CAD build for the part. Positions are in the model's coordinates, mm. Face numbers are marked on the shaded views. Give positions to 0.01 mm unless a question says otherwise; leave off trailing zeros. Loops run counter-clockwise (first coordinate to the right, second up) from the corner with the lowest first, then second, coordinate; pieces in that order, holes last.
```python
from build123d import *

# Parameters (mm, degrees)
SKETCH1_R                = 6.35
BOSS_EXTRUDE1_DEPTH      = 25.4
F_0_257_DIAMETER_HOLE1_D = 6.5278
CHAMFER1_SIZE            = 0.4


with BuildPart() as part:
    # Sketch1 → Boss-Extrude1 (new body)
    with BuildSketch(Plane.XY):
        Circle(SKETCH1_R)
    extrude(amount=BOSS_EXTRUDE1_DEPTH)

    # F (0.257) Diameter Hole1 (through all)
    with Locations(Plane.XY.offset(25.4)):
        with Locations((0, 0)):
            Hole(F_0_257_DIAMETER_HOLE1_D / 2)

    # Chamfer1
    chamfer1_edges = [part.edges().sort_by_distance(p)[0] for p in [
        (3.2639, 0, 25.4),
        (3.2639, 0, 0),
    ]]
    chamfer(chamfer1_edges, length=CHAMFER1_SIZE)


solid = part.part
```
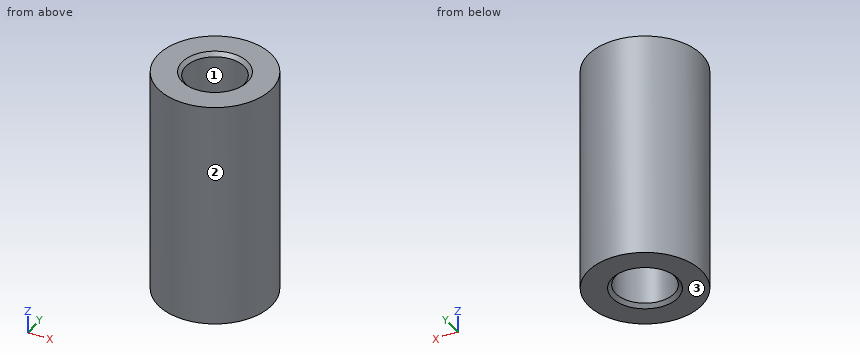
1. Probe line 1 along Y through (x, z) = (0, 19); line 2 along X through (y, z) = (1.75, 12.25); line 3 along X through (y, z) = (2.75, 24.5). List the from-to ranges inside material, lowest first.
Responses:
line 1: y = -6.35 to -3.26, 3.26 to 6.35
line 2: x = -6.1 to -2.76, 2.76 to 6.1
line 3: x = -5.72 to -1.76, 1.76 to 5.72
2. Pull direction Y, two halves, no side cores. Call the marked faces 1, 2 and 3: released by +Y, released by -Y, zero draft, split by the parting line, or undercut.
Responses:
face 1: undercut
face 2: split by the parting line
face 3: zero draft
3. Saw through at A-A, the plane y = 0. List the corners of the cut face in (x, z), and give its area (3 significant figures).
Responses:
outline: (-6.35, 0) - (-3.66, 0) - (-3.26, 0.4) - (-3.26, 25) - (-3.66, 25.4) - (-6.35, 25.4) - close; (3.26, 0.4) - (3.66, 0) - (6.35, 0) - (6.35, 25.4) - (3.66, 25.4) - (3.26, 25) - close
area: 156 mm2
4. Saw through at D-D, the plane y = -4.75. List the corners of the cut face in (x, z), and give its area (3 significant figures).
Responses:
outline: (-4.21, 0) - (4.21, 0) - (4.21, 25.4) - (-4.21, 25.4) - close
area: 214 mm2
5. Drop flat-ended pins along their axis: pin 1 (3 mm diameter, centred on y = -4.5, z = 20.5, fed in from -X); pin 2 (3 mm diameter, centred on x = 4, z = 18, fed in from +Y). Give the stop position or say it passes through.
Responses:
pin 1: stops at x = -5.6
pin 2: stops at y = 5.84
6. Saw through at C-C, the plane z = 19.75. List the corners of the cut face in (x, y).
Responses:
outline: circle Ø12.7 at (0, 0); hole circle Ø6.53 at (0, 0)
